Source: three-view drawing plus pictorial views. Frame: mm from the lowest corner of the part. Give positions to 0.01 mm unless a question says otherwise; leave off trailing zeros. Order: outer loops, then holes, each group sorted by start corner. A loop starts at its lowest first (then second) coordinate and runs counter-clockwise, first axis right, second up. Notation, with made-up numbers: (73.5, 86.5) - (116.5, 86.5) arc R29 ccw to (116.5, 107.5) - close; hole circle Ø6 at (37.5, 17). An arc over 180 degrees is marked (long way). Answer in a Markdown table with one row per item. Add a question column.
1. Contact query for a flat-ended pin moving along its axis: pin 1 (0.5 mm diameter, centred on y = 33, z = 0.5, fed in from -X). Output: stop coordinate, or through.
2. Ray query, line 1 (Y direction, x = 17, z = 0.8); line 2 (X direction, y = 11.5, z = 0.65); line 3 (Y direction, x = 53, z = 0.85). Return the intervals inside material, ascending. Write a range as [from, to].
3. Section query A-A on x = 17.5. Return loops of the section in (y, z), and give its area (3 significant figures).
4. Section query C-C on y = 15. Return loops of the section in (x, z).
5. Section query B-B on z = 0.85. Return loops of the section in (x, y).
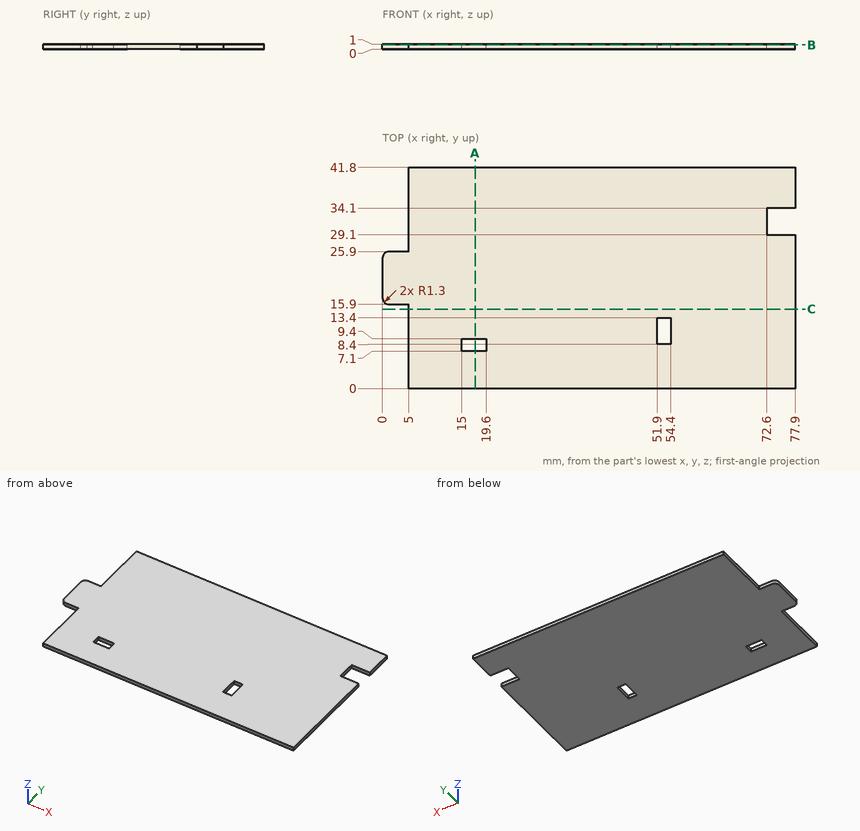
Answer:
| question | item | result |
|---|---|---|
| 1 | pin 1 | stops at x = 5 |
| 2 | line 1 | y = [0, 7.1], [9.4, 41.8] |
| 2 | line 2 | x = [5, 51.9], [54.4, 77.9] |
| 2 | line 3 | y = [0, 8.4], [13.4, 41.8] |
| 3 | outline | (0, 0) - (7.1, 0) - (7.1, 1) - (0, 1) - close; (9.4, 0) - (41.8, 0) - (41.8, 1) - (9.4, 1) - close |
| 3 | area | 39.5 mm² |
| 4 | outline | (5, 0) - (77.9, 0) - (77.9, 1) - (5, 1) - close |
| 5 | outline | (0, 17.2) arc R1.3 ccw to (1.3, 15.9) - (5, 15.9) - (5, 0) - (77.9, 0) - (77.9, 29.1) - (72.6, 29.1) - (72.6, 34.1) - (77.9, 34.1) - (77.9, 41.8) - (5, 41.8) - (5, 25.9) - (1.3, 25.9) arc R1.3 ccw to (0, 24.6) - close; hole (15, 7.1) - (19.6, 7.1) - (19.6, 9.4) - (15, 9.4) - close; hole (51.9, 8.4) - (54.4, 8.4) - (54.4, 13.4) - (51.9, 13.4) - close |
